Autodesk Inventor part; units mm, degrees
ref_plane "YZ Plane" through (0, 0, 0) normal (1, 0, 0) x (0, 1, 0)
ref_plane "XZ Plane" through (0, 0, 0) normal (0, 1, 0) x (-1, 0, 0)
ref_plane "XY Plane" through (0, 0, 0) normal (0, 0, 1) x (1, 0, 0)
sketch "Sketch1" plane through (0, 0, 0) normal (0, 0, 1) x (1, 0, 0)
  line L0 (0, 0) -> (42, 0)
  line L1 (42, 0) -> (42, 70)
  line L2 (42, 70) -> (0, 70)
  line L3 (0, 70) -> (0, 0)
  line L4 (31.75, 14.25) -> (10.25, 14.25)
  line L5 (10.25, 14.25) -> (10.25, 55.75)
  line L6 (10.25, 55.75) -> (31.75, 55.75)
  line L7 (31.75, 55.75) -> (31.75, 14.25)
  line L8 (31.75, 14.25) -> (10.25, 55.75) construction
  line L9 (10.25, 14.25) -> (31.75, 55.75) construction
  line L10 (21, 70) -> (21, 0)
  line L11 (0, 35) -> (42, 35)
  point P0 (21, 35)
  point P1 (10.8, 7)
  point P2 (31.2, 7)
  point P3 (31.2, 0)
  point P4 (10.8, 0)
  point P5 (31.75, 35)
  point P6 (21, 35)
  point P7 (10.25, 35)
  point P8 (21, 14.25)
  point P9 (21, 55.75)
  dimension "d0" = 42
  dimension "d1" = 70
  dimension "d4" = 21.5
  dimension "d5" = 41.5
extrude "Extrusion1" add sketch "Sketch1" along normal blind 2
fillet "Fillet3" radius 3 2 edges at (42, 70, 1) (0, 70, 1)
extrude "Extrusion11" cut sketch "Sketch1" along normal blind 6 contours L10 L11 L7 L4 | L4 L5 L11 L10 | L5 L6 L10 L11 | L10 L6 L7 L11
sketch "Sketch14" plane through (0, 0, 2) normal (0, 0, 1) x (1, 0, 0)
  line L0 (31.75, 55.75) -> (10.25, 55.75)
  circle A0 centre (16.15, 59.2) radius 2.15
  circle A1 centre (25.85, 59.2) radius 2.15
  line L1 (16.15, 59.2) -> (25.85, 59.2)
  line L2 (10.8, 35) -> (31.2, 35)
  circle A2 centre (16.15, 10.8) radius 2.15
  circle A3 centre (25.85, 10.8) radius 2.15
  line L3 (16.15, 10.8) -> (25.85, 10.8)
  line L4 (0, 0) -> (42, 0)
  arc A4 (3, 70) -> (0, 67) centre (3, 67) ccw
  line L5 (0, 67) -> (0, 0)
  line L6 (42, 0) -> (42, 67)
  arc A5 (42, 67) -> (39, 70) centre (39, 67) ccw
  line L7 (39, 70) -> (3, 70)
  point P0 (21, 59.2)
  dimension "d54" = 4.3
  dimension "d55" = 4.3
  dimension "d56" = 9.7
extrude "Extrusion12" cut sketch "Sketch14" against normal blind 6 contours A0 | A1 | A2 | A3
sketch "Sketch17" plane through (0, 0, 2) normal (0, 0, 1) x (1, 0, 0)
  circle A0 centre (16.15, 10.8) radius 2.15
  circle A1 centre (25.85, 59.2) radius 2.15
  circle A2 centre (25.85, 10.8) radius 2.15
  circle A3 centre (16.15, 59.2) radius 2.15
  line L0 (10.25, 55.75) -> (31.75, 55.75)
  line L1 (31.75, 55.75) -> (31.75, 14.25)
  line L2 (31.75, 14.25) -> (10.25, 14.25)
  line L3 (10.25, 14.25) -> (10.25, 55.75)
  circle A4 centre (16.15, 59.2) radius 2.15
  circle A5 centre (25.85, 59.2) radius 2.15
  line L4 (16.15, 61.35) -> (25.85, 61.35)
  line L5 (25.85, 59.2) -> (25.85, 61.35)
  line L6 (14, 59.2) -> (14, 55.75)
  line L7 (28, 59.2) -> (28, 55.75)
  line L8 (10.25, 55.75) -> (10.25, 14.25)
  line L9 (10.25, 55.75) -> (10.25, 62.75)
  line L10 (10.25, 62.75) -> (31.75, 62.75)
  line L11 (31.75, 62.75) -> (31.75, 55.75)
  line L12 (0, 0) -> (42, 0)
  arc A6 (3, 70) -> (0, 67) centre (3, 67) ccw
  line L13 (0, 67) -> (0, 0)
  line L14 (42, 0) -> (42, 67)
  arc A7 (42, 67) -> (39, 70) centre (39, 67) ccw
  line L15 (39, 70) -> (3, 70)
  dimension "d67" = 7
extrude "Extrusion15" add sketch "Sketch17" along normal blind 2 contours L7 L0 L6 A3 L4 A1 | A1 L4 A3 L6 L0 L9 L10 L11 L7
sketch "Sketch18" plane through (0, 0, 2) normal (0, 0, 1) x (1, 0, 0)
  line L0 (10.25, 14.25) -> (10.25, 55.75)
  line L1 (10.25, 62.75) -> (31.75, 62.75)
  line L2 (31.75, 55.75) -> (31.75, 14.25)
  line L3 (31.75, 14.25) -> (10.25, 14.25)
  circle A0 centre (25.85, 10.8) radius 2.15
  circle A1 centre (16.15, 10.8) radius 2.15
  line L4 (10.25, 40.625) -> (5.625, 40.625)
  line L5 (5.625, 40.625) -> (5.625, 69)
  circle A2 centre (5.625, 40.625) radius 1.5
  line L6 (21, 80.706) -> (21, -3.1342)
  circle A3 centre (36.375, 40.625) radius 1.5
  line L7 (0, 0) -> (42, 0)
  arc A4 (3, 70) -> (0, 67) centre (3, 67) ccw
  line L8 (0, 67) -> (0, 0)
  line L9 (42, 0) -> (42, 67)
  arc A5 (42, 67) -> (39, 70) centre (39, 67) ccw
  line L10 (39, 70) -> (3, 70)
  line L11 (10.25, 55.75) -> (10.25, 62.75)
  line L12 (31.75, 62.75) -> (31.75, 55.75)
  dimension "d70" = 4.625
  dimension "d71" = 28.375
  dimension "d72" = 3
  dimension "d75" = 30.75
extrude "Extrusion16" cut sketch "Sketch18" against normal blind 10 contours A2 L5 L4 | L4 L5 A2 | A3
sketch "Sketch22" plane through (0, 0, 2) normal (0, 0, 1) x (1, 0, 0)
  point P0 (0, 0)
sketch "Sketch23" plane through (0, 0, 4) normal (0, 0, 1) x (1, 0, 0)
  line L0 (31.75, 55.75) -> (31.75, 62.75)
  line L1 (31.75, 62.75) -> (10.25, 62.75)
  line L2 (10.25, 62.75) -> (10.25, 55.75)
  line L3 (10.25, 55.75) -> (31.75, 55.75)
  circle A0 centre (25.85, 59.2) radius 2.15
  circle A1 centre (16.15, 59.2) radius 2.15
  line L4 (10.5, 56) -> (10.5, 62.5)
  line L5 (10.5, 62.5) -> (31.5, 62.5)
  line L6 (31.5, 62.5) -> (31.5, 56)
  line L7 (31.5, 56) -> (10.5, 56)
  point P0 (0, 0)
  dimension "d88" = 0.25
extrude "Extrusion20" cut sketch "Sketch23" against normal blind 2 contours L3 L2 L1 L0
sketch "Sketch24" plane through (0, 0, 2) normal (0, 0, 1) x (1, 0, 0)
  line L0 (10.5, 62.5) -> (10.5, 56)
  line L1 (31.5, 62.5) -> (10.5, 62.5)
  line L2 (31.5, 56) -> (31.5, 62.5)
  line L3 (10.5, 56) -> (31.5, 56)
  circle A0 centre (5.625, 40.625) radius 1.5
  circle A1 centre (36.375, 40.625) radius 1.5
  arc A2 (3, 70) -> (0, 67) centre (3, 67) ccw
  line L4 (0, 67) -> (0, 0)
  line L5 (0, 0) -> (42, 0)
  line L6 (42, 0) -> (42, 67)
  arc A3 (42, 67) -> (39, 70) centre (39, 67) ccw
  line L7 (39, 70) -> (3, 70)
  line L8 (31.75, 55.75) -> (10.25, 55.75)
  line L9 (31.75, 55.75) -> (31.75, 14.25)
  line L10 (31.75, 14.25) -> (10.25, 14.25)
  line L11 (10.25, 14.25) -> (10.25, 55.75)
  circle A4 centre (25.85, 10.8) radius 2.15
  circle A5 centre (16.15, 10.8) radius 2.15
  line L12 (42, 14.25) -> (0, 14.25)
  line L13 (0, 14.25) -> (0, 0)
  line L14 (0, 0) -> (42, 0)
  line L15 (42, 0) -> (42, 14.25)
  point P0 (31.75, 14.25)
extrude "Extrusion21" cut sketch "Sketch24" against normal blind 10 contours L12 L10 L6 L5 L4
properties part number "MG995_26_upgrade_3DPrint"
Can you work these out from the model? Positions are in its coordinate system, mm. A direction names the side the tool comes from. Give positions to 0.01 mm unless a question says otherwise; leave off trailing zeros. Loops run counter-clockwise (first coordinate to the right, second up) from the corner with the lowest first, then second, coordinate; pieces in that order, holes last. Notation, with made-up numbers: M 67,6 L 113,6 A34 cw 113,44 Z; hole C 9,10.5 d3. An arc over 180 degrees is marked long. Use CSV: the item, a comma, the result in double quotes. Start each with the question number.
1. Imagine slicing it at A-A, the plane y = 53. Write out the boundary of the cut face in (x, z).
2. If we mould it in two halves opening along Y, with no side actions, what happens to faces 5 (the face through (5, 14.25, 1)), 6 (the face through (21, 59, 4)), 7 (the face through (5.3, 39.16, 1.01)), 8 (the face through (0.9, 69.14, 1.01))? For each: released by +Y, released by -Y, zero draft, split by the parting line, or undercut.
3. Imagine slicing it at B-B, the plane x = 16.15. Write out the boundary of the cut face in (y, z), plus the area to 3 significant figures.
4. For P1, Ø8, axis at x = 9.5, y = 31.5, coming from the +Z side; P2, Ø1.6, axis at x = 26, z = 1.5, coming from the -Y side; P3, Ø0.6, axis at x = 20, z = 2.5, coming from the -Y side, each with a flat end and sliding along its axis, tell me the tip position at first contact or that it passes through.
5. Imagine slicing it at D-D, the plane y = 59.2. Write out the boundary of the cut face in (x, z).
6. On a 3-axis mill with a long thin cutter (end or side, diameter ignored), from which of +Z, -Z, +X, -X, +Y, -Y can I reach the whole of each face in a straight line? I mean faces 1 (the face through (10.5, 59, 3)), 2 (the face through (21, 62.5, 3)), 3 (the face through (31.5, 59, 3)), 4 (the face through (31.75, 35, 1)). Say none if no direction works.
7. Imagine slicing it at C-C, the plane z = 3.1. Write out the boundary of the cut face in (x, y), plus the area to 3 significant figures.
8. If I drill on L1, parallel to X at y = 59.2, z = 1.8; L2, parallel to X at y = 28.5, z = 0.5; L3, parallel to X at y = 60.5, z = 1.3, over which ranges is the centre line in solid material (lowest first)?
Response values:
1,outline,"M 0,0 L 10.25,0 L 10.25,2 L 0,2 Z; M 31.75,0 L 42,0 L 42,2 L 31.75,2 Z"
2,face 5,"released by -Y"
2,face 6,"zero draft"
2,face 7,"undercut"
2,face 8,"released by +Y"
3,outline,"M 55.75,0 L 57.05,0 L 57.05,4 L 56,4 L 56,2 L 55.75,2 Z; M 61.35,0 L 70,0 L 70,2 L 62.5,2 L 62.5,4 L 61.35,4 Z"
3,area,"24.3 mm^2"
4,P1,"z = 2"
4,P2,"y = 55.75"
4,P3,"y = 56"
5,outline,"M 0,0 L 14,0 L 14,4 L 10.5,4 L 10.5,2 L 0,2 Z; M 18.3,0 L 23.7,0 L 23.7,4 L 18.3,4 Z; M 28,0 L 42,0 L 42,2 L 31.5,2 L 31.5,4 L 28,4 Z"
6,face 1,"+Z, -X, +Y, -Y"
6,face 2,"+Z, +X, -X, +Y"
6,face 3,"+Z, +X, +Y, -Y"
6,face 4,"+Z, -Z, -Y"
7,outline,"M 10.5,56 L 31.5,56 L 31.5,62.5 L 10.5,62.5 Z; hole C 16.15,59.2 d4.3; hole C 25.85,59.2 d4.3"
7,area,"107 mm^2"
8,L1,"0 to 14, 18.3 to 23.7, 28 to 42"
8,L2,"0 to 10.25, 31.75 to 42"
8,L3,"0 to 14.44, 17.86 to 24.14, 27.56 to 42"
